Design review of the part shown in the three views and the two pictorial views. Dimensions are in mm from the part's minimum x, y and z. Round coordinates to 2 decimals unless told otherwise and drop trailing zeros. Order: outer loops, then holes, each group sorted by start corner. A loop starts at its lowest first (then second) coordinate and runs counter-clockwise, first axis right, second up. Notation, with made-up numbers: M 68.5,73.5 L 75.5,73.5 A10 cw 75.5,87.5 Z; hole C 28,5.25 d11. An arc over 180 degrees is marked long. Write each question's results on one line, items separated by ' | '. Start each with the question number.
Item 1: Take a section at A-A, the plane y = 5.08. Write out the cut boundary in (x, z), plus the area to 3 significant figures.
Item 2: Take a section at C-C, the plane y = 160.02. Write out the cut boundary in (x, z), plus the area to 3 significant figures.
Item 3: Clearance check with flat-ended pins moving along their axes: pin 1 (4 mm diameter, centred on x = 121, y = 41.5, fed in from +Z); pin 2 (3 mm diameter, centred on y = 84, z = 3.5, fed in from -X). State where each tip first meets the part, or that it passes through.
Item 4: Take a section at D-D, the plane x = 146. Write out the cut boundary in (y, z).
Item 5: Wall thickness on line 1 (Y direction, x = 6.99, z = 2.4); line 2 (Y direction, x = 164.47, z = 3.75); line 3 (Z direction, x = 13, y = 107): over which ranges is each line inside the solid? List them lowest first. Write a range as [from, to].
Item 6: Take a section at B-B, the plane x = 164.47. Write out the cut boundary in (y, z).
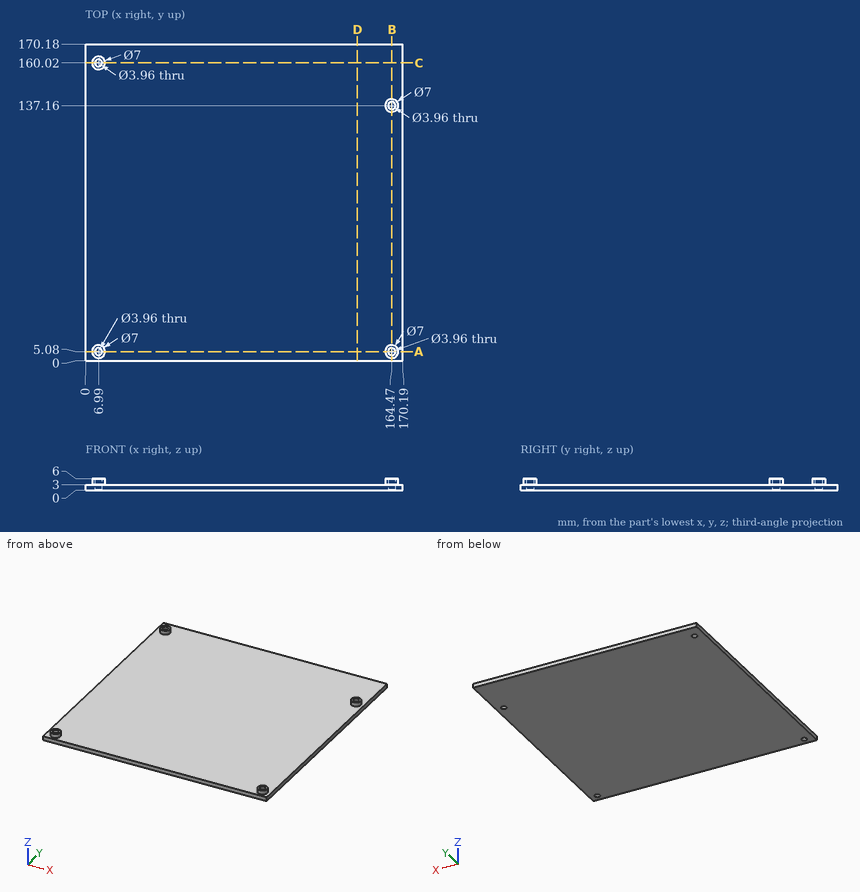
Results list:
1) outline: M 0,0 L 5.01,0 L 5.01,6 L 3.49,6 L 3.49,3 L 0,3 Z; M 8.97,0 L 162.49,0 L 162.49,6 L 160.97,6 L 160.97,3 L 10.49,3 L 10.49,6 L 8.97,6 Z; M 166.45,0 L 170.19,0 L 170.19,3 L 167.97,3 L 167.97,6 L 166.45,6 Z | area: 505 mm²
2) outline: M 0,0 L 5.01,0 L 5.01,6 L 3.49,6 L 3.49,3 L 0,3 Z; M 8.97,0 L 170.19,0 L 170.19,3 L 10.49,3 L 10.49,6 L 8.97,6 Z | area: 508 mm²
3) pin 1: z = 3 | pin 2: x = 0
4) outline: M 0,0 L 170.18,0 L 170.18,3 L 0,3 Z
5) line 1: [0, 3.1], [7.06, 158.04], [162, 170.18] | line 2: [1.58, 3.1], [7.06, 8.58], [133.66, 135.18], [139.14, 140.66] | line 3: [0, 3]
6) outline: M 0,0 L 3.1,0 L 3.1,6 L 1.58,6 L 1.58,3 L 0,3 Z; M 7.06,0 L 135.18,0 L 135.18,6 L 133.66,6 L 133.66,3 L 8.58,3 L 8.58,6 L 7.06,6 Z; M 139.14,0 L 170.18,0 L 170.18,3 L 140.66,3 L 140.66,6 L 139.14,6 Z
